For this review, take the finished solid that the model builds, in its own axes (mm). Round coordinates to 2 decimals unless told otherwise and drop trailing zeros. Order: outer loops, then holes, each group sorted by start corner. A loop starts at its lowest first (then second) coordinate and runs counter-clockwise, first axis right, second up. Notation, with made-up numbers: (6.5, -17.5) -> (36.5, -17.5) arc R27 ccw to (36.5, 4.5) -> close; hole circle Ø11 at (6, 42). An arc over 180 degrees is marked (long way). Use a Markdown table: item, result. Add a question column.
1) Clearance check with flat-ended pins moving along their axes: P1, Ø1, axis at y = -77, z = 2, coming from the -X side; P2, Ø1.6, axis at y = 77.5, z = 1, coming from the +X side; P3, Ø1.5, axis at y = -2.5, z = 2.5, coming from the +X side. State where each tip first meets the part, or that it passes through.
2) Draft analysis for pull direction Y (two halves, no side actions). For faces 1 (the face through (-0.759, 11.583, 1.612)), 2 (the face through (1, 1, 3.18)), state which applies: pulls with the +Y half, pulls with the -Y half, needs draft (parallel to the pull), parting line crosses it, or undercut.
3) Consider section C-C (x = 34). State the section outline as (y, z) points, plus the area to 3 significant figures.
4) Wall thickness on line 1 along Y through (x, z) = (13.75, 1.2); line 2 along X through (y, z) = (76.59, 1.8); line 3 along X through (y, z) = (2, 0.2): over which ranges is each line inside the solid? List them lowest first. Write a range as [from, to].
5) Consider section A-A (y = 43.7). State the section outline as (x, z) points.
6) Consider section B-B (y = 15). State the section outline as (x, z) points.
```python
from build123d import *

# Parameters (mm, degrees)
SKETCH1_R           = 1.5
BOSS_EXTRUDE1_DEPTH = 3.18
SKETCH2_R           = 1.5
SKETCH2_R_2         = 3.5
CUT_EXTRUDE1_DEPTH  = 10
SKETCH3_R           = 3.656100146
CUT_EXTRUDE2_DEPTH  = 10


with BuildPart() as part:
    # Sketch1 → Boss-Extrude1 (new body)
    with BuildSketch(Plane.XY):
        Polygon((-78.18, 75), (-12.5, 75), (-12.5, 78.18), (12.5, 78.18), (12.5, 75), (78.18, 75), (78.18, 12.5), (75, 12.5), (75, 1.5), (71, 1.5), (71, 4.5), (68, 4.5), (68, 1.5), (65.18, 1.5), (65.18, -1.5), (68, -1.5), (68, -4.5), (71, -4.5), (71, -1.5), (75, -1.5), (75, -12.5), (78.18, -12.5), (78.18, -75), (12.5, -75), (12.5, -78.18), (-12.5, -78.18), (-12.5, -75), (-78.18, -75), (-78.18, -12.5), (-75, -12.5), (-75, -1.5), (-71, -1.5), (-71, -4.5), (-68, -4.5), (-68, -1.5), (-65.18, -1.5), (-65.18, 1.5), (-68, 1.5), (-68, 4.5), (-71, 4.5), (-71, 1.5), (-75, 1.5), (-75, 12.5), (-78.18, 12.5), align=None)
        with Locations(Location((0, -76.59, 0), (0, 0, 180))):
            Circle(SKETCH1_R, mode=Mode.SUBTRACT)
        with Locations(Location((0, 76.59, 0), (0, 0, 180))):
            Circle(SKETCH1_R, mode=Mode.SUBTRACT)
    extrude(amount=BOSS_EXTRUDE1_DEPTH)

    # Sketch2 → Cut-Extrude1 (cut)
    with BuildSketch(Plane.XY.offset(3.18)):
        with Locations((-13.75, -4.3)):
            Circle(SKETCH2_R)
        with Locations((0, -25.8)):
            Circle(SKETCH2_R)
        with Locations((13.75, -4.3)):
            Circle(SKETCH2_R)
        with Locations((0, 4.2)):
            Circle(SKETCH2_R)
        with Locations((13.75, 25.7)):
            Circle(SKETCH2_R)
        with Locations((-13.75, 25.7)):
            Circle(SKETCH2_R)
        with Locations((0, 15)):
            Circle(SKETCH2_R_2)
        with Locations((0, -15)):
            Circle(SKETCH2_R_2)
    extrude(amount=-CUT_EXTRUDE1_DEPTH, mode=Mode.SUBTRACT)

    # Sketch3 → Cut-Extrude2 (cut)
    with BuildSketch(Plane(origin=(0, 0, 0), x_dir=(-1, 0, 0), z_dir=(0, 0, -1))):
        with Locations((1e-09, 43.7)):
            Circle(SKETCH3_R)
    extrude(amount=-CUT_EXTRUDE2_DEPTH, mode=Mode.SUBTRACT)


solid = part.part
```
Results list:
| question | item | result |
|---|---|---|
| 1 | P1 | x = -12.5 |
| 1 | P2 | x = 12.5 |
| 1 | P3 | x = 75 |
| 2 | face 1 | undercut |
| 2 | face 2 | needs draft |
| 3 | outline | (-75, 0) -> (75, 0) -> (75, 3.18) -> (-75, 3.18) -> close |
| 3 | area | 477 mm2 |
| 4 | line 1 | [-75, -5.8], [-2.8, 24.2], [27.2, 75] |
| 4 | line 2 | [-12.5, -1.5], [1.5, 12.5] |
| 4 | line 3 | [-75, -71], [-68, 68], [71, 75] |
| 5 | outline | (-78.18, 0) -> (-3.66, 0) -> (-3.66, 3.18) -> (-78.18, 3.18) -> close; (3.66, 0) -> (78.18, 0) -> (78.18, 3.18) -> (3.66, 3.18) -> close |
| 6 | outline | (-78.18, 0) -> (-3.5, 0) -> (-3.5, 3.18) -> (-78.18, 3.18) -> close; (3.5, 0) -> (78.18, 0) -> (78.18, 3.18) -> (3.5, 3.18) -> close |
